```python
from build123d import *

# Parameters (mm, degrees)
SKETCH1_R           = 53.975
SKETCH1_R_2         = 47.625
BOSS_EXTRUDE1_DEPTH = 8.89
BOSS_EXTRUDE2_START = -44.45
SKETCH1_4_R         = 53.975
SKETCH1_4_R_2       = 47.625
BOSS_EXTRUDE2_DEPTH = 44.45
CUT_EXTRUDE1_DEPTH  = 25.4
BOSS_EXTRUDE3_START = 3.4925
SKETCH3_R           = 47.625
SKETCH3_R_2         = 34.925
BOSS_EXTRUDE3_DEPTH = 3.4925
SKETCH4_R           = 1.5
CUT_EXTRUDE2_DEPTH  = 21.2725


with BuildPart() as part:
    # Sketch1 → Boss-Extrude1 (new body)
    # profile 1 of 2: a face of its own
    with BuildSketch(Plane(origin=(0, 0, 0), x_dir=(1, 0, 0), z_dir=(0, 1, 0))):
        with Locations(Location((0, 0, 0), (0, 0, 270))):
            Circle(SKETCH1_R)
        Circle(SKETCH1_R_2, mode=Mode.SUBTRACT)
    # profile 2 of 2: a face of its own
    with BuildSketch(Plane(origin=(0, 0, 0), x_dir=(1, 0, 0), z_dir=(0, 1, 0))):
        Circle(SKETCH1_R_2)
    extrude(amount=BOSS_EXTRUDE1_DEPTH)

    # Sketch1_4 → Boss-Extrude2 (add)
    with BuildSketch(Plane(origin=(0, 0, 0), x_dir=(1, 0, 0), z_dir=(0, 1, 0)).offset(BOSS_EXTRUDE2_START)):
        with Locations(Location((0, 0, 0), (0, 0, 270))):
            Circle(SKETCH1_4_R)
        with Locations(Location((0, 0, 0), (0, 0, 270))):
            Circle(SKETCH1_4_R_2, mode=Mode.SUBTRACT)
    extrude(amount=BOSS_EXTRUDE2_DEPTH)

    # Sketch2 → Cut-Extrude1 (cut)
    with BuildSketch(Plane(origin=(0, 8.89, 0), x_dir=(1, 0, 0), z_dir=(0, 1, 0))):
        with BuildLine():
            Line((-2, 1.5), (2, 1.5))
            ThreePointArc((2, 1.5), (2.5, 0), (2, -1.5))
            Line((2, -1.5), (-2, -1.5))
            ThreePointArc((-2, -1.5), (-2.5, 0), (-2, 1.5))
        make_face()
    extrude(amount=-CUT_EXTRUDE1_DEPTH, mode=Mode.SUBTRACT)

    # Sketch3 → Boss-Extrude3 (add)
    with BuildSketch(Plane.XZ.offset(BOSS_EXTRUDE3_START)):
        with Locations(Location((0, 0, 0), (0, 0, 90))):
            Circle(SKETCH3_R)
        with Locations(Location((0, 0, 0), (0, 0, 270))):
            Circle(SKETCH3_R_2, mode=Mode.SUBTRACT)
    extrude(amount=-BOSS_EXTRUDE3_DEPTH)

    # Sketch4 → Cut-Extrude2 (cut)
    with BuildSketch(Plane(origin=(0, 8.89, 0), x_dir=(1, 0, 0), z_dir=(0, 1, 0))):
        with Locations(Location((25.4, 0, 0), (0, 0, 270))):
            Circle(SKETCH4_R)
        with Locations(Location((-25.4, 0, 0), (0, 0, 270))):
            Circle(SKETCH4_R)
    extrude(amount=-CUT_EXTRUDE2_DEPTH, mode=Mode.SUBTRACT)


solid = part.part
```
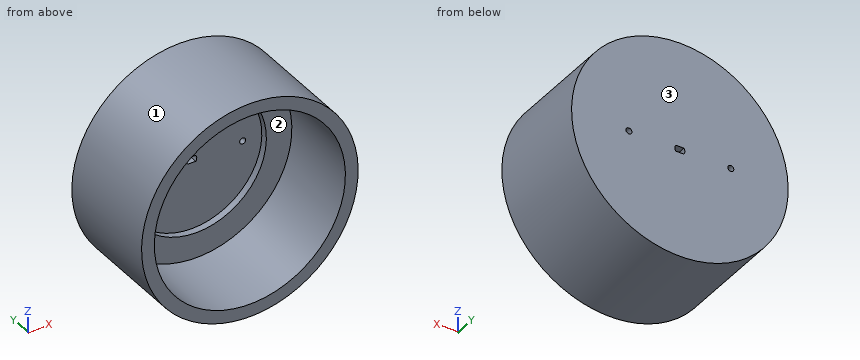
Verification items for the finished model (mm, model axes). Face numbers are marked on the shaded views. Give positions to 0.01 mm unless a question says otherwise; leave off trailing zeros. Write each loop counter-clockwise with the first axis right and the second up, starting at its lowest first coordinate (ties: lowest second). Pieces come first, ordered by that corner, then holes. Notation, with made-up numbers: (27, -16) - (56, -16) arc R28 cw to (56, 11) - close; hole circle Ø9 at (41.25, -31.75). An arc over 180 degrees is marked (long way). Put each result on its own line as item: value.
Q1. Mould release check, pull along X, two halves, no side actions. Record for the marked faces 1, 2 and 3: released by +X, released by -X, zero draft, split by the parting line, or undercut.
Result:
face 1: split by the parting line
face 2: undercut
face 3: zero draft
Q2. Section check D-D on y = -2. Record the cut outline in (x, z) (3 decimals).
Result:
outline: circle Ø107.95 at (0, 0); hole circle Ø69.85 at (0, 0)
Q3. Section check C-C on z = 0. Count the separate pieces of the cut face and the enclosed holes in it, and give its area (3 significant figures).
Result:
separate pieces: 4
enclosed holes: 0
area: 1,520 mm2
Q4. Section check B-B on y = 4. Record the cut outline in (x, z) (3 decimals).
Result:
outline: circle Ø107.95 at (0, 0); hole circle Ø3 at (-25.4, 0); hole (-2, -1.5) - (2, -1.5) arc R2.5 ccw to (2, 1.5) - (-2, 1.5) arc R2.5 ccw to start; hole circle Ø3 at (25.4, 0)
Q5. Scan lines: probe 1 along X at (y, z) = (2, 0) (3 decimals); probe 2 along Y at (x, z) = (21.5, 32); probe 3 along Y at (x, z) = (6.5, 20). Record each from-to range of solid material in increasing order. Write a range as from..to.
Result:
probe 1: -53.975..-26.9, -23.9..-2.5, 2.5..23.9, 26.9..53.975
probe 2: -3.49..8.89
probe 3: 0..8.89
Q6. Depth check by flat-ended pin: P1, Ø8, axis at x = -28, y = -25.5, coming from the +Z side; P2, Ø2, axis at x = -1.5, z = 38.5, coming from the -Y side; P3, Ø5, axis at x = -25.4, z = 0, coming from the -Y side; P4, Ø2.5, axis at x = 25.4, z = 0, coming from the +Y side. Enter the tip coordinate at first touch or a pass-through.
Result:
P1: z = 48.35
P2: y = -3.49
P3: y = 0
P4: through
